from build123d import *

# Parameters (mm, degrees)
F1_DEPTH = 12.7
F0_R     = 6.35
F2_DEPTH = 25.4
F3_DEPTH = 38.1
F4_R     = 6.35
F5_R     = 6.35
F6_DEPTH = 25.4


with BuildPart() as f1:
    # F0 (on Front) → F1 (new body)
    with BuildSketch(Plane.XZ):
        with BuildLine():
            Line((-25.4, 12.7), (25.4, 12.7))
            ThreePointArc((25.4, 12.7), (16.419744, 16.419744), (12.7, 25.4))
            Line((12.7, 25.4), (12.7, 57.15))
            ThreePointArc((12.7, 57.15), (0, 44.45), (-12.7, 57.15))
            Line((-12.7, 57.15), (-12.7, 25.4))
            ThreePointArc((-12.7, 25.4), (-16.419744, 16.419744), (-25.4, 12.7))
        make_face()
    extrude(amount=F1_DEPTH)

    # F0 (on Front) → F2 (join)
    with BuildSketch(Plane.XZ):
        with BuildLine():
            ThreePointArc((-12.7, 57.15), (0, 44.45), (12.7, 57.15))
            ThreePointArc((12.7, 57.15), (0, 69.85), (-12.7, 57.15))
        make_face()
        with Locations((0, 57.15)):
            Circle(F0_R, mode=Mode.SUBTRACT)
    extrude(amount=F2_DEPTH)

    # F0 (on Front) → F3 (join)
    with BuildSketch(Plane.XZ):
        Polygon((-25.4, 0), (0, 0), (25.4, 0), (25.4, 12.7), (-25.4, 12.7), align=None)
    extrude(amount=F3_DEPTH)

    # F4
    f4_edges = [f1.edges().sort_by_distance(p)[0] for p in [
        (-25.4, -38.1, 6.35),
        (25.4, -38.1, 6.35),
    ]]
    fillet(f4_edges, radius=F4_R)

    # F5 (on face) → F6 (cut)
    with BuildSketch(Plane(origin=(0, 0, 0), x_dir=(1, 0, 0), z_dir=(0, 0, -1))):
        with Locations((0, 25.4)):
            Circle(F5_R)
    extrude(amount=-F6_DEPTH, mode=Mode.SUBTRACT)


solid = f1.part
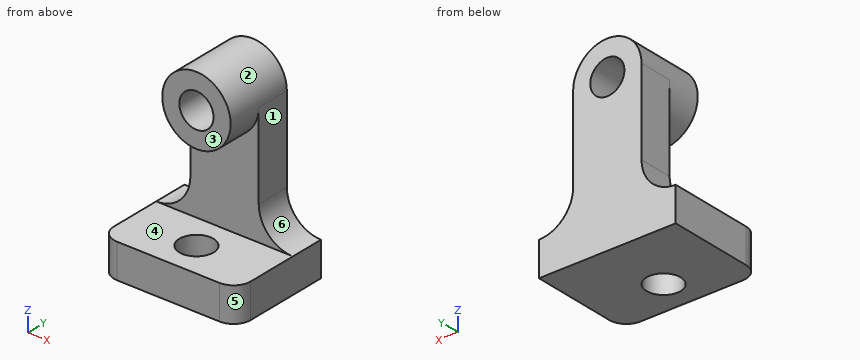
Model file for the job. Use its own axes, mm. Face numbers are marked on the shaded views. A direction names the side the tool comes from. Coordinates: 2 decimals unless noted, no trailing zeros. Loops run counter-clockwise (first coordinate to the right, second up) from the corner with the lowest first, then second, coordinate; pieces in that order, holes last. Notation, with made-up numbers: (57.5, 60.25) -> (96.5, 60.25) arc R30 cw to (96.5, 85.25) -> close; hole circle Ø11 at (-24.5, 13.5). An arc over 180 degrees is marked (long way). Use one line per item in the form item = value. Start each with the question number.
(1) Probe probe 1 along Z at (x, y) = (0, -15.25); probe 2 along X at (y, z) = (-25.4, 10.25); probe 3 along Z at (x, y) = (0, -5.75). List the from-to ranges inside material, lowest first. Write a range as from..to.
(2) Cut at C-C on z = 10. Give the cut face in (x, y).
(3) Cut at D-D on y = -14. Give the cut face in (x, z).
(4) Tool access for the marked faces 1, 2 and 3: list every direction of +Z, -Z, +X, -X, +Y, -Y with a clear straight run to the whole face (end or side of a thin tool).
(5) Flat gauge pins, fed straight in: pin 1 (4 mm diameter, centred on x = -12.5, z = 30.5, fed in from -Y); pin 2 (10 mm diameter, centred on y = -9, z = 37.5, fed in from -X); pin 3 (20.5 mm diameter, centred on x = 0, z = 57.15, fed in from -Y). Where does each tip first touch, or does it go through?
(6) Cut at B-B on y = -6.5. Give the cut face in (x, z), and give its area (3 significant figures).
(7) Pull direction Z, two halves, no side cores. Call the marked faces 4, 5 and 6: pulls with the +Z half, pulls with the -Z half, needs draft (parallel to the pull), parting line crosses it, or undercut.
(8) Cut at A-A on x = 0. Give the cut face in (y, z), and give its area (3 significant figures).
Values:
q1.probe_1 = 0..12.7, 44.45..50.8, 63.5..69.85
q1.probe_2 = -25.4..-6.35, 6.35..25.4
q1.probe_3 = 0..50.8, 63.5..69.85
q2.outline = (-25.4, -31.75) arc R6.35 ccw to (-19.05, -38.1) -> (19.05, -38.1) arc R6.35 ccw to (25.4, -31.75) -> (25.4, 0) -> (-25.4, 0) -> close; hole circle Ø12.7 at (0, -25.4)
q3.outline = (-25.4, 0) -> (25.4, 0) -> (25.4, 12.7) -> (-25.4, 12.7) -> close; circle Ø25.4 at (0, 57.15); hole circle Ø12.7 at (0, 57.15)
q4.face_1 = +Z, +X, +Y, -Y
q4.face_2 = -Y
q4.face_3 = +Z, +X, -X, -Y
q5.pin_1 = -12.7
q5.pin_2 = -12.7
q5.pin_3 = -25.4
q6.outline = (-25.4, 0) -> (25.4, 0) -> (25.4, 12.7) arc R12.7 cw to (12.7, 25.4) -> (12.7, 57.15) arc R12.7 ccw to (-12.7, 57.15) -> (-12.7, 25.4) arc R12.7 cw to (-25.4, 12.7) -> close; hole circle Ø12.7 at (0, 57.15)
q6.area = 1,970 mm2
q7.face_4 = undercut
q7.face_5 = needs draft
q7.face_6 = pulls with the +Z half
q8.outline = (-38.1, 0) -> (-31.75, 0) -> (-31.75, 12.7) -> (-38.1, 12.7) -> close; (-25.4, 44.45) -> (-12.7, 44.45) -> (-12.7, 12.7) -> (-19.05, 12.7) -> (-19.05, 0) -> (0, 0) -> (0, 50.8) -> (-25.4, 50.8) -> close; (-25.4, 63.5) -> (0, 63.5) -> (0, 69.85) -> (-25.4, 69.85) -> close
q8.area = 1,050 mm2
